```python
from build123d import *

# Parameters (mm, degrees)
EXTRUDE1_DEPTH = 74.93
SKETCH2_R      = 1.905
EXTRUDE2_DEPTH = 3.175
SKETCH3_W      = 37.880364804
SKETCH3_H      = 3.00059593
EXTRUDE3_DEPTH = 15.24
FILLET1_R      = 2.54
FILLET2_R      = 0.762
EXTRUDE4_DEPTH = 17.78
SKETCH5_W      = 39.584129336
SKETCH5_H      = 3.52111337
EXTRUDE5_DEPTH = 17.78


with BuildPart() as part:
    # Sketch1 → Extrude1 (new body)
    with BuildSketch(Plane.XY):
        with BuildLine():
            Line((2.54, 0), (48.26, 0))
            ThreePointArc((48.26, 0), (50.056051224, 0.743948776), (50.8, 2.54))
            Line((50.8, 2.54), (50.8, 13.97))
            ThreePointArc((50.8, 13.97), (50.056051224, 15.766051224), (48.26, 16.51))
            Line((48.26, 16.51), (2.54, 16.51))
            ThreePointArc((2.54, 16.51), (0.743948776, 15.766051224), (0, 13.97))
            Line((0, 13.97), (0, 2.54))
            ThreePointArc((0, 2.54), (0.743948776, 0.743948776), (2.54, 0))
        make_face()
    extrude(amount=-EXTRUDE1_DEPTH)

    # Sketch2 → Extrude2 (add)
    with BuildSketch(Plane(origin=(0, 0, 0), x_dir=(0, 0, -1), z_dir=(1, 0, 0))):
        with Locations((9.525, 7.112)):
            Circle(SKETCH2_R)
    extrude2 = extrude(amount=-EXTRUDE2_DEPTH)

    # Mirror1: Extrude2 across plane
    add(extrude2.mirror(Plane(origin=(25.4, 0, 0), x_dir=(0, 0, 1), z_dir=(1, 0, 0))))

    # Sketch3 → Extrude3 (add)
    with BuildSketch(Plane.XY):
        with Locations((25.4, 9.017)):
            Rectangle(SKETCH3_W, SKETCH3_H)
    extrude(amount=EXTRUDE3_DEPTH)

    # Fillet1
    fillet1_edges = [part.edges().sort_by_distance(p)[0] for p in [
        (44.340182402, 9.017, 15.24),
        (6.459817598, 9.017, 15.24),
    ]]
    fillet(fillet1_edges, radius=FILLET1_R)

    # Fillet2
    fillet2_edges = [part.edges().sort_by_distance(p)[0] for p in [
        (44.340182402, 9.017, 0),
        (25.4, 10.517297965, 0),
        (6.459817598, 9.017, 0),
        (25.4, 7.516702035, 0),
    ]]
    fillet(fillet2_edges, radius=FILLET2_R)

    # Sketch4 → Extrude4 (cut)
    with BuildSketch(Plane(origin=(0, 10.517297965, 0), x_dir=(-1, 0, 0), z_dir=(0, 1, 0))):
        with BuildLine():
            Line((-36.179236435, 10.183663009), (-14.620763565, 10.183663009))
            ThreePointArc((-14.620763565, 10.183663009), (-12.457260283, 8.020159727), (-14.620763565, 5.856656445))
            Line((-14.620763565, 5.856656445), (-36.179236435, 5.856656445))
            ThreePointArc((-36.179236435, 5.856656445), (-38.342739717, 8.020159727), (-36.179236435, 10.183663009))
        make_face()
    extrude(amount=-EXTRUDE4_DEPTH, mode=Mode.SUBTRACT)

    # Sketch5 → Extrude5 (cut)
    with BuildSketch(Plane(origin=(0, 0, -74.93), x_dir=(-1, 0, 0), z_dir=(0, 0, -1))):
        with Locations((-25.4, 8.255)):
            Rectangle(SKETCH5_W, SKETCH5_H)
    extrude(amount=-EXTRUDE5_DEPTH, mode=Mode.SUBTRACT)


solid = part.part
```
Part model, mm, in its own coordinate system. A direction names the side the tool comes from. Give positions to 0.01 mm unless a question says otherwise; leave off trailing zeros. Loops run counter-clockwise (first coordinate to the right, second up) from the corner with the lowest first, then second, coordinate; pieces in that order, holes last. Notation, with made-up numbers: M 39.5,37 L 62.5,37 A16 ccw 62.5,67 Z; hole C 35.25,-30 d8. An arc over 180 degrees is marked long. Return JSON: item names as keys, results as strings.
1) Saw through at D-D, the plane z = 7. List the corners of the cut face in (x, y), then the cut area to 3 significant figures.
Calculated:
{"outline": "M 6.46,7.52 L 12.71,7.52 L 12.71,10.52 L 6.46,10.52 Z; M 38.09,7.52 L 44.34,7.52 L 44.34,10.52 L 38.09,10.52 Z", "area": "37.5 mm2"}
2) Saw through at C-C, the plane z = -69. List the corners of the cut face in (x, y), then the cut area to 3 significant figures.
Calculated:
{"outline": "M 0,2.54 A2.54 ccw 2.54,0 L 48.26,0 A2.54 ccw 50.8,2.54 L 50.8,13.97 A2.54 ccw 48.26,16.51 L 2.54,16.51 A2.54 ccw 0,13.97 Z; hole M 5.61,6.49 L 45.19,6.49 L 45.19,10.02 L 5.61,10.02 Z", "area": "694 mm2"}
3) Drill centre lines: line 1 (Y direction, x = 33.5, z = -57.5); line 2 (Z direction, x = 29, y = 9.5); line 3 (X direction, y = 2.75, z = -50.5). Where is each one in solid material? Low to high.
Calculated:
{"line 1": "y = 0 to 6.49, 10.02 to 16.51", "line 2": "z = -57.15 to 5.86, 10.18 to 15.24", "line 3": "x = 0 to 50.8"}
4) Flat gauge pins, fed straight in: pin 1 Ø1.5 at (x, y) = (21.5, 6) entering from +Z; pin 2 Ø0.9 at (y, z) = (9, 6) entering from -X; pin 3 Ø1.5 at (x, y) = (30, 9.5) entering from -Z; pin 4 Ø1.1 at (y, z) = (9, -68) entering from -X. Where does each tip first touch, or does it go through?
Calculated:
{"pin 1": "stops at z = 0", "pin 2": "stops at x = 6.46", "pin 3": "stops at z = -74.93", "pin 4": "stops at x = 0"}
5) Saw through at B-B, the plane z = -16.5. List the corners of the cut face in (x, y).
Calculated:
{"outline": "M 0,2.54 A2.54 ccw 2.54,0 L 48.26,0 A2.54 ccw 50.8,2.54 L 50.8,13.97 A2.54 ccw 48.26,16.51 L 2.54,16.51 A2.54 ccw 0,13.97 Z"}
6) Pull direction X, two halves, no side cores. Call faces 4 (the face through (25, 0, -37)), 5 (the face through (38.342, 9.038, 7.973)), 6 (the face through (50.036, 0.724, -36.94)): released by +X, released by -X, zero draft, split by the parting line, or undercut.
Calculated:
{"face 4": "zero draft", "face 5": "undercut", "face 6": "released by +X"}
7) 3-axis set-ups, long thin cutter, end or side, ignore diameter. For faces 1 (the face through (26, 6.494, -66)), 2 (the face through (52.365, 5.953, -8.013)), 3 (the face through (25, 10.517, 11)): which of +Z, -Z, +X, -X, +Y, -Y reach the whole face in a straight line?
Calculated:
{"face 1": "-Z", "face 2": "+X", "face 3": "+Z, +X, -X, +Y"}
8) Saw through at A-A, the plane x = 26.5. List the corners of the cut face in (y, z), then the cut area to 3 significant figures.
Calculated:
{"outline": "M 0,-74.93 L 6.49,-74.93 L 6.49,-57.15 L 10.02,-57.15 L 10.02,-74.93 L 16.51,-74.93 L 16.51,0 L 11.28,0 A0.76 cw 10.52,0.76 L 10.52,5.86 L 7.52,5.86 L 7.52,0.76 A0.76 cw 6.75,0 L 0,0 Z; M 7.52,10.18 L 10.52,10.18 L 10.52,15.24 L 7.52,15.24 Z", "area": "1,210 mm2"}
